```python
from build123d import *

# Parameters (mm, degrees)
EXTRUDE_1_DEPTH      = 15
EXTRUDE_1_DEPTH_BACK = 15
FILLET_4_R           = 1
SKETCH_2_R           = 1.1
CUT_EXTRUDE_1_DEPTH  = 10
SKETCH_3_R           = 1.703478165
CUT_EXTRUDE_2_DEPTH  = 10


with BuildPart() as part:
    # Sketch 1 → Extrude 1 (new, two sides: drawn at the far end of the back side and taken through both)
    with BuildSketch(Plane(origin=(0, 0, 0), x_dir=(0, 0, -1), z_dir=(1, 0, 0)).offset(-EXTRUDE_1_DEPTH_BACK)):
        with BuildLine():
            Line((-67.5, 3), (-67.5, 1))
            Line((-67.5, 1), (-62.961481397, 1))
            ThreePointArc((-62.961481397, 1), (-50, 13), (-37.038518603, 1))
            Line((-37.038518603, 1), (-35.038518603, 1))
            Line((-35.038518603, 1), (-35.038518603, 7))
            Line((-35.038518603, 7), (35.038518603, 7))
            Line((35.038518603, 7), (35.038518603, 1))
            Line((35.038518603, 1), (37.038518603, 1))
            ThreePointArc((37.038518603, 1), (50, 13), (62.961481397, 1))
            Line((62.961481397, 1), (67.5, 1))
            Line((67.5, 1), (67.5, 3))
            Line((67.5, 3), (64.696938457, 3))
            ThreePointArc((64.696938457, 3), (53.289128952, 14.634945533), (38, 9))
            Line((38, 9), (-38, 9))
            ThreePointArc((-38, 9), (-53.289128952, 14.634945533), (-64.696938457, 3))
            Line((-64.696938457, 3), (-67.5, 3))
        make_face()
    extrude(amount=EXTRUDE_1_DEPTH + EXTRUDE_1_DEPTH_BACK)

    # Fillet 4
    fillet_4_edges = [part.edges().sort_by_distance(p)[0] for p in [
        (0, 7, 35.038518603),
        (0, 7, -35.038518603),
    ]]
    fillet(fillet_4_edges, radius=FILLET_4_R)

    # Sketch 2 → Cut-Extrude 1 (cut, symmetric)
    with BuildSketch(Plane(origin=(0, 3, 0), x_dir=(1, 0, 0), z_dir=(0, 1, 0))):
        with Locations(Location((0, 65.5, 0), (0, 0, 90))):
            Circle(SKETCH_2_R)
    cut_extrude_1 = extrude(amount=CUT_EXTRUDE_1_DEPTH, both=True, mode=Mode.SUBTRACT)

    # Sketch 3 → Cut-Extrude 2 (cut)
    with BuildSketch(Plane(origin=(0, 3, 0), x_dir=(1, 0, 0), z_dir=(0, 1, 0))):
        with Locations((0, 65.5)):
            Circle(SKETCH_3_R)
    cut_extrude_2 = extrude(amount=CUT_EXTRUDE_2_DEPTH, mode=Mode.SUBTRACT)

    # Mirror 1: Cut-Extrude 1, Cut-Extrude 2 across plane
    add(cut_extrude_1.mirror(Plane.XY), mode=Mode.SUBTRACT)
    add(cut_extrude_2.mirror(Plane.XY), mode=Mode.SUBTRACT)


solid = part.part
```
CAD build for the part. Positions are in the model's coordinates, mm. A direction names the side the tool comes from. Coordinates: 2 decimals unless noted, no trailing zeros. Order: outer loops, then holes, each group sorted by start corner. A loop starts at its lowest first (then second) coordinate and runs counter-clockwise, first axis right, second up. Notation, with made-up numbers: (81, 59) - (138, 59) arc R25 cw to (138, 86) - close; hole circle Ø5 at (75.25, 75.25). An arc over 180 degrees is marked (long way). Answer in a Markdown table with one row per item.
1. Slice it at B-B, the plane z = 57.5. List the corners of the cut face in (x, y).
Answer:
| item | result |
|---|---|
| outline | (-15, 10.62) - (15, 10.62) - (15, 12.99) - (-15, 12.99) - close |
2. Flat gauge pins, fed straight in: P1, Ø6, axis at x = -10, y = 7, coming from the +Z side; P2, Ø1.5, axis at x = 9.5, z = 18.5, coming from the +Y side; P3, Ø1.9, axis at x = 5, z = -66, coming from the +Y side. Where does each tip first touch, or does it go through?
Answer:
| item | result |
|---|---|
| P1 | z = 64.46 |
| P2 | y = 9 |
| P3 | y = 3 |
3. Slice it at C-C, the plane z = -20. List the corners of the cut face in (x, y), then the cut area to 3 significant figures.
Answer:
| item | result |
|---|---|
| outline | (-15, 7) - (15, 7) - (15, 9) - (-15, 9) - close |
| area | 60.0 mm² |
4. 3-axis set-ups, long thin cutter, end or side, ignore diameter. For faces 5 (the face through (0, 9, -1)), 6 (the face through (15, 8.6, 5.3)), 7 (the face through (0, 7, 0)): which of +Z, -Z, +X, -X, +Y, -Y reach the whole face in a straight line?
Answer:
| item | result |
|---|---|
| face 5 | +X, -X, +Y |
| face 6 | +Z, -Z, +X, +Y, -Y |
| face 7 | +X, -X, -Y |
5. Slice it at A-A, the plane x = 11.5. List the corners of the cut face in (y, z).
Answer:
| item | result |
|---|---|
| outline | (1, -67.5) - (3, -67.5) - (3, -64.7) arc R15 ccw to (9, -38) - (9, 38) arc R15 ccw to (3, 64.7) - (3, 67.5) - (1, 67.5) - (1, 62.96) arc R13 cw to (1, 37.04) - (1, 35.04) - (6, 35.04) arc R1 cw to (7, 34.04) - (7, -34.04) arc R1 cw to (6, -35.04) - (1, -35.04) - (1, -37.04) arc R13 cw to (1, -62.96) - close |
6. Pull direction Z, two halves, no side cores. Call faces 1 (the face through (-0.026, 4.102, 63.797)), 2 (the face through (0, 13, 50)), 3 (the face through (-0.026, 4.102, -63.797)), 4 (the face through (0, 3, -67)): +Z half, -Z half, draft (parallel to the pull), parting line (faces both ways), or undercut.
Answer:
| item | result |
|---|---|
| face 1 | +Z half |
| face 2 | undercut |
| face 3 | -Z half |
| face 4 | draft |
7. Drill centre lines: L1, parallel to X at y = 1.8, z = -65.5; L2, parallel to Z at x = -11.5, y = 6; L3, parallel to Z at x = 2.5, y = 6.25. Where is each one in solid material? Low to high. Write a range as from..to.
Answer:
| item | result |
|---|---|
| L1 | -15..-1.1, 1.1..15 |
| L2 | -63.75..-61.53, -38.47..-35.04, 35.04..38.47, 61.53..63.75 |
| L3 | -63.64..-61.4, -38.6..-35.01, 35.01..38.6, 61.4..63.64 |
